Source: three-view drawing plus pictorial views. Frame: mm from the lowest corner of the part. A direction names the side the tool comes from. Coordinates: 2 decimals unless noted, no trailing zeros. Write each loop counter-clockwise with the first axis right and the second up, starting at its lowest first coordinate (ties: lowest second). Pieces come first, ordered by that corner, then holes. Notation, with made-up numbers: (-11, -10) -> (39, -10) arc R21 ccw to (39, 25) -> close; hole circle Ø6 at (-34.75, 45). An arc over 180 degrees is marked (long way). One line per item, written item: value.
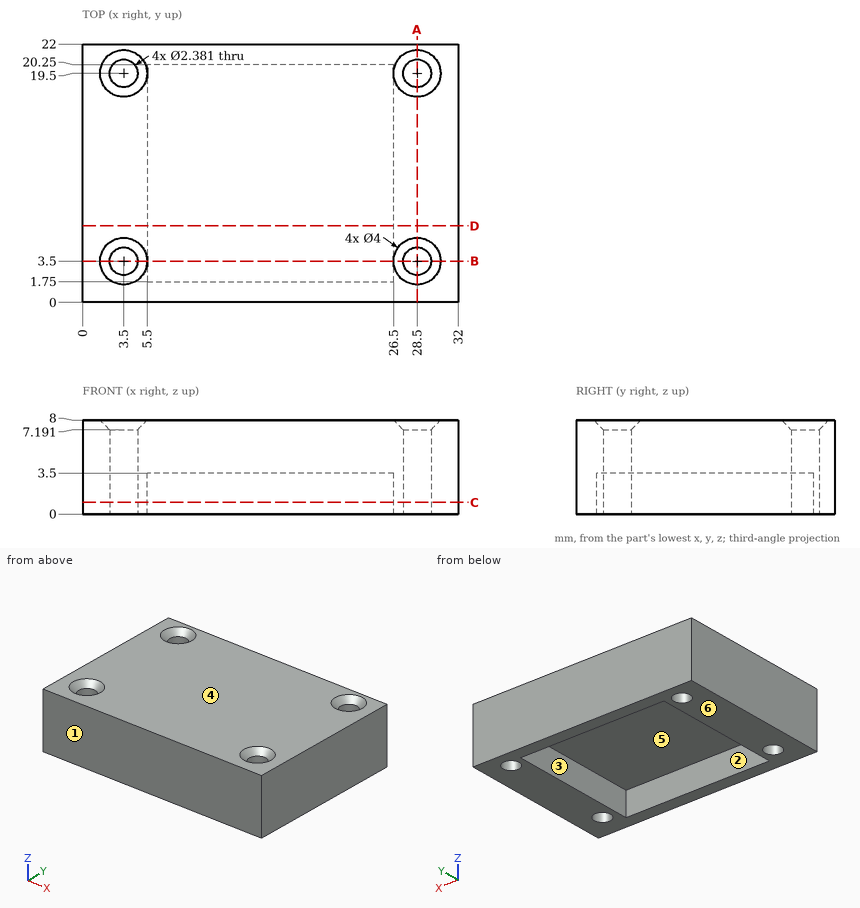
(1) Section D-D (y = 6.5). Return the cut outline in (x, z).
Responses:
outline: (0, 0) -> (5.5, 0) -> (5.5, 3.5) -> (26.5, 3.5) -> (26.5, 0) -> (32, 0) -> (32, 8) -> (0, 8) -> close
(2) Reachability of the marked faces 5 and 6 from +Z, -Z, +X, -X, +Y, -Y: full face, straight path, thin tool, end or side. Return the list, or none.
Responses:
face 5: -Z
face 6: -Z, +X, -X, +Y, -Y
(3) Line query: line 1 (X direction, y = 19.5, z = 3); line 2 (X direction, y = 3.5, z = 5); line 3 (Y direction, x = 18, z = 1.5). Output: solid intervals per line, ascending. Write a range as [from, to].
Responses:
line 1: x = [0, 2.31], [4.69, 5.5], [26.5, 27.31], [29.69, 32]
line 2: x = [0, 2.31], [4.69, 27.31], [29.69, 32]
line 3: y = [0, 1.75], [20.25, 22]
(4) Section A-A (x = 28.5). Return the cut outline in (y, z), then the cut area to 3 significant figures.
Responses:
outline: (0, 0) -> (2.31, 0) -> (2.31, 7.19) -> (1.5, 8) -> (0, 8) -> close; (4.69, 0) -> (18.31, 0) -> (18.31, 7.19) -> (17.5, 8) -> (5.5, 8) -> (4.69, 7.19) -> close; (20.69, 0) -> (22, 0) -> (22, 8) -> (21.5, 8) -> (20.69, 7.19) -> close
area: 137 mm2
(5) Section B-B (y = 3.5). Return the cut outline in (x, z).
Responses:
outline: (0, 0) -> (2.31, 0) -> (2.31, 7.19) -> (1.5, 8) -> (0, 8) -> close; (4.69, 0) -> (5.5, 0) -> (5.5, 3.5) -> (26.5, 3.5) -> (26.5, 0) -> (27.31, 0) -> (27.31, 7.19) -> (26.5, 8) -> (5.5, 8) -> (4.69, 7.19) -> close; (29.69, 0) -> (32, 0) -> (32, 8) -> (30.5, 8) -> (29.69, 7.19) -> close
(6) Pull-direction query (Y, two-part tool) for the marked faces 1, 2, 3 and 4; classes: released by +Y, released by -Y, zero draft, split by the parting line, or undercut.
Responses:
face 1: released by -Y
face 2: undercut
face 3: undercut
face 4: zero draft
(7) Section C-C (z = 1). Return the cut outline in (x, y), then the cut area to 3 significant figures.
Responses:
outline: (0, 0) -> (32, 0) -> (32, 22) -> (0, 22) -> close; hole circle Ø2.38 at (3.5, 3.5); hole circle Ø2.38 at (3.5, 19.5); hole (5.5, 1.75) -> (26.5, 1.75) -> (26.5, 20.25) -> (5.5, 20.25) -> close; hole circle Ø2.38 at (28.5, 3.5); hole circle Ø2.38 at (28.5, 19.5)
area: 298 mm2
(8) First-contact query: pin 1 (4 mm diameter, centred on x = 18.5, z = 1, fed in from -Y); pin 2 (1.9 mm diameter, centred on x = 28.5, y = 19.5, fed in from -Z); pin 3 (1 mm diameter, centred on x = 12.5, y = 3, fed in from -Z). Flat tips, straight axial feed; report the tip coordinate or a pass-through.
Responses:
pin 1: stops at y = 0
pin 2: passes through
pin 3: stops at z = 3.5
